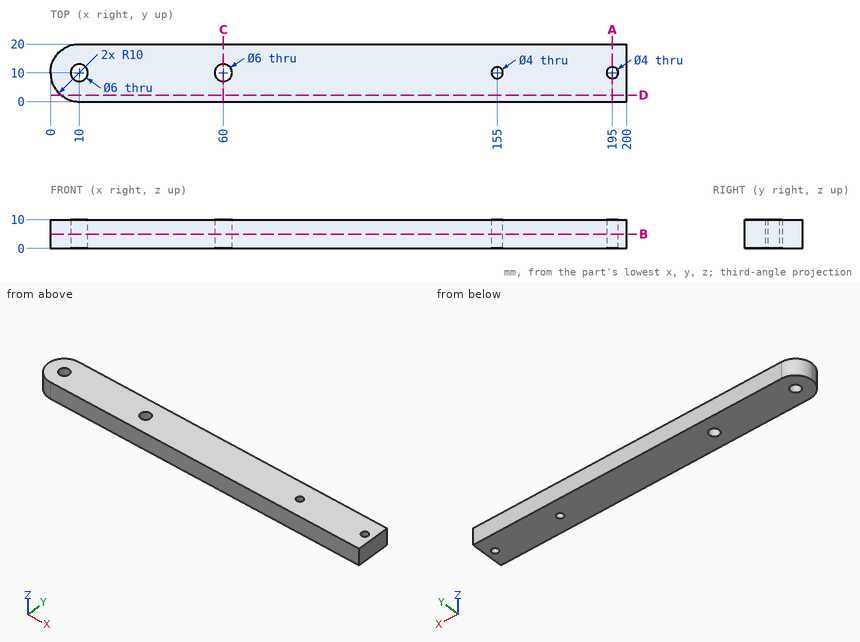
Check sheet for the drawn part. Datum: minimum x, y, z corner. Units: mm. Round coordinates to 2 decimals unless told otherwise and drop trailing zeros. Loops run counter-clockwise (first coordinate to the right, second up) from the corner with the lowest first, then second, coordinate; pieces in that order, holes last. Notation, with made-up numbers: M -11.5,25 L -5.5,25 A21 cw -5.5,58 Z; hole C 87,22.25 d9. An arc over 180 degrees is marked long. One line per question, with ' | ' between items. Start each with the question number.
Item 1: Scan lines: probe 1 along X at (y, z) = (8.25, 5.75) (1 decimal); probe 2 along X at (y, z) = (8.5, 1.25); probe 3 along X at (y, z) = (16.75, 2.25). Record each from-to range of solid material in increasing order.
Item 2: Section check C-C (x = 60). Record the boundary of the cut face in (y, z).
Item 3: Section check A-A (x = 195). Record the boundary of the cut face in (y, z).
Item 4: Section check B-B (z = 5). State how many separate pieces and enclosed holes the cut face has, and give its area (3 significant figures).
Item 5: Section check D-D (y = 2.25). Record the boundary of the cut face in (x, z).
Worked out:
1) probe 1: 0.2 to 7.6, 12.4 to 57.6, 62.4 to 154, 156 to 194, 196 to 200 | probe 2: 0.11 to 7.4, 12.6 to 57.4, 62.6 to 153.68, 156.32 to 193.68, 196.32 to 200 | probe 3: 2.62 to 200
2) outline: M 0,0 L 7,0 L 7,10 L 0,10 Z; M 13,0 L 20,0 L 20,10 L 13,10 Z
3) outline: M 0,0 L 8,0 L 8,10 L 0,10 Z; M 12,0 L 20,0 L 20,10 L 12,10 Z
4) separate pieces: 1 | enclosed holes: 4 | area: 3,880 mm^2
5) outline: M 3.68,0 L 200,0 L 200,10 L 3.68,10 Z
